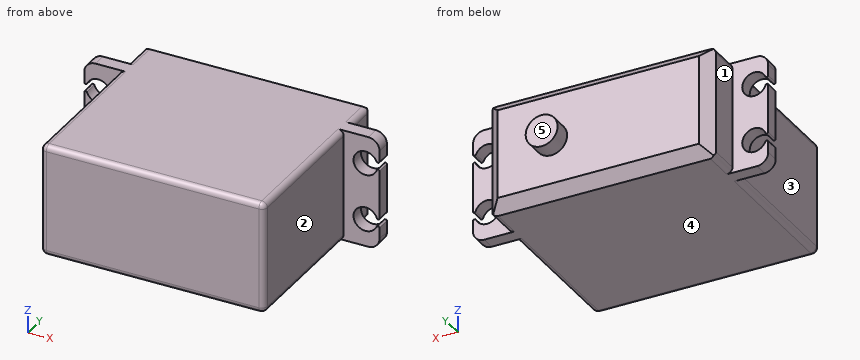
```python
from build123d import *

# Parameters (mm, degrees)
SKETCH_1_W           = 40
SKETCH_1_H           = 20
EXTRUDE_1_DEPTH      = 36.5
SKETCH_2_W           = 52.8
SKETCH_2_H           = 20
EXTRUDE_2_DEPTH      = 2.5
SKETCH_3_R           = 2.15
CUT_EXTRUDE_1_DEPTH  = 4.15
SKETCH_4_W           = 1.589858097
SKETCH_4_H           = 1.269072198
CUT_EXTRUDE_2_DEPTH  = 4.15
FILLET_2_R           = 2
FILLET_3_R           = 1
FILLET_7_R           = 0.2
FILLET_8_R           = 0.2
FILLET_START         = 38.537319575
FILLET_3_2_OUTLINE_W = 42
FILLET_3_2_OUTLINE_H = 6
FILLET_3_2_DEPTH     = 2.462680425
FILLET_START_2       = 24.395183951
FILLET_4_OUTLINE_W   = 42
FILLET_4_OUTLINE_H   = 6
FILLET_4_DEPTH       = 2.604816049
FILLET_START_3       = 52.679455198
FILLET_5_OUTLINE_W   = 5
FILLET_5_OUTLINE_H   = 22
FILLET_5_DEPTH       = 2.320544802
FILLET_START_4       = -27
FILLET_6_OUTLINE_W   = 6
FILLET_6_OUTLINE_H   = 22
FILLET_6_DEPTH       = 2.604816049
SKETCH_5_R           = 2.85
EXTRUDE_3_DEPTH      = 5
CUT_EXTRUDE_START    = -1.8
SKETCH_6_R           = 2.85
CUT_EXTRUDE_3_DEPTH  = 1.8


with BuildPart() as part:
    # 草图1 → 凸台-拉伸1 (new body)
    with BuildSketch(Plane(origin=(0, 0, 0), x_dir=(1, 0, 0), z_dir=(0, 1, 0))):
        with Locations((20, 10)):
            Rectangle(SKETCH_1_W, SKETCH_1_H)
    extrude(amount=EXTRUDE_1_DEPTH)

    # 草图2 → 凸台-拉伸2 (add)
    with BuildSketch(Plane(origin=(0, 26.5, 0), x_dir=(-1, 0, 0), z_dir=(0, -1, 0))):
        with Locations((-20, 10)):
            Rectangle(SKETCH_2_W, SKETCH_2_H)
    extrude(amount=-EXTRUDE_2_DEPTH)

    # 草图3 → 切除-拉伸1 (cut)
    with BuildSketch(Plane(origin=(0, 29, 0), x_dir=(1, 0, 0), z_dir=(0, 1, 0))):
        with Locations(Location((43.9, 15.1, 0), (0, 0, 270))):
            Circle(SKETCH_3_R)
        with Locations(Location((43.9, 4.9, 0), (0, 0, 270))):
            Circle(SKETCH_3_R)
        with Locations(Location((-3.9, 15.1, 0), (0, 0, 270))):
            Circle(SKETCH_3_R)
        with Locations(Location((-3.9, 4.9, 0), (0, 0, 270))):
            Circle(SKETCH_3_R)
    extrude(amount=-CUT_EXTRUDE_1_DEPTH, mode=Mode.SUBTRACT)

    # 草图4 → 切除-拉伸2 (cut)
    with BuildSketch(Plane(origin=(0, 29, 0), x_dir=(1, 0, 0), z_dir=(0, 1, 0))):
        with Locations((-6.117219692, 15.174989867)):
            Rectangle(SKETCH_4_W, SKETCH_4_H)
        with Locations((46.117219692, 15.174989867)):
            Rectangle(SKETCH_4_W, SKETCH_4_H)
        with Locations((46.117219692, 4.825010133)):
            Rectangle(SKETCH_4_W, SKETCH_4_H)
        with Locations((-6.117219692, 4.825010133)):
            Rectangle(SKETCH_4_W, SKETCH_4_H)
    extrude(amount=-CUT_EXTRUDE_2_DEPTH, mode=Mode.SUBTRACT)

    # 圆角2
    fillet_2_edges = [part.edges().sort_by_distance(p)[0] for p in [
        (46.4, 27.75, -20),
        (-6.4, 27.75, 0),
        (46.4, 27.75, 0),
        (-6.4, 27.75, -20),
    ]]
    fillet(fillet_2_edges, radius=FILLET_2_R)

    # Fillet 3
    fillet_3_edges = [part.edges().sort_by_distance(p)[0] for p in [
        (0, 13.25, -20),
        (40, 13.25, -20),
        (40, 13.25, 0),
        (0, 13.25, 0),
        (20, 0, -20),
        (40, 0, -10),
        (20, 0, 0),
        (0, 0, -10),
        (0, 32.75, -20),
        (40, 32.75, -20),
        (40, 32.75, 0),
        (0, 32.75, 0),
    ]]
    fillet(fillet_3_edges, radius=FILLET_3_R)

    # 圆角7
    fillet_7_edges = [part.edges().sort_by_distance(p)[0] for p in [
        (46.4, 27.75, -4.190474034),
        (46.4, 27.75, -5.459546232),
        (45.97591137, 27.75, -5.459546232),
        (45.929549926, 27.75, -4.190474034),
        (45.97591137, 27.75, -14.540453768),
        (45.929549926, 27.75, -15.809525966),
        (-5.97591137, 27.75, -5.459546232),
        (-5.929549926, 27.75, -4.190474034),
        (46.4, 27.75, -15.809525966),
        (46.4, 27.75, -14.540453768),
        (-6.4, 27.75, -4.190474034),
        (-6.4, 27.75, -5.459546232),
    ]]
    fillet(fillet_7_edges, radius=FILLET_7_R)

    # 圆角8
    fillet_8_edges = [part.edges().sort_by_distance(p)[0] for p in [
        (-6.4, 27.75, -14.540453768),
        (-6.4, 27.75, -15.809525966),
        (-5.929549926, 27.75, -15.809525966),
        (-5.97591137, 27.75, -14.540453768),
    ]]
    fillet(fillet_8_edges, radius=FILLET_8_R)

    # Fillet 3 2: read off the stored shape, not the designer's step
    # Fillet 3 2 outline → Fillet 3 2 (cut)
    with BuildSketch(Plane(origin=(0, 0, 0), x_dir=(1, 0, 0), z_dir=(0, 0.707106781186547, -0.707106781186548)).offset(FILLET_START)):
        with Locations((20, -12)):
            Rectangle(FILLET_3_2_OUTLINE_W, FILLET_3_2_OUTLINE_H)
    extrude(amount=FILLET_3_2_DEPTH, mode=Mode.SUBTRACT)

    # 倒角4: read off the stored shape, not the designer's step
    # 倒角4 outline → 倒角4 (cut)
    with BuildSketch(Plane(origin=(0, 0, 0), x_dir=(1, 0, 0), z_dir=(0, 0.707106781186547, 0.707106781186548)).offset(FILLET_START_2)):
        with Locations((20, 26)):
            Rectangle(FILLET_4_OUTLINE_W, FILLET_4_OUTLINE_H)
    extrude(amount=FILLET_4_DEPTH, mode=Mode.SUBTRACT)

    # 倒角5: read off the stored shape, not the designer's step
    # 倒角5 outline → 倒角5 (cut)
    with BuildSketch(Plane(origin=(0, 0, 0), x_dir=(0.707106781186546, -0.707106781186549, 0), z_dir=(0.707106781186549, 0.707106781186546, 0)).offset(FILLET_START_3)):
        with Locations((2.5, 10)):
            Rectangle(FILLET_5_OUTLINE_W, FILLET_5_OUTLINE_H)
    extrude(amount=FILLET_5_DEPTH, mode=Mode.SUBTRACT)

    # 倒角6: read off the stored shape, not the designer's step
    # 倒角6 outline → 倒角6 (cut)
    with BuildSketch(Plane(origin=(0, 0, 0), x_dir=(0.7071067811865471, 0.707106781186548, 0), z_dir=(0.707106781186548, -0.707106781186547, 0)).offset(FILLET_START_4)):
        with Locations((26, -10)):
            Rectangle(FILLET_6_OUTLINE_W, FILLET_6_OUTLINE_H)
    extrude(amount=FILLET_6_DEPTH, mode=Mode.SUBTRACT)

    # 草图5 → 凸台-拉伸3 (add)
    with BuildSketch(Plane(origin=(0, 36.5, 0), x_dir=(1, 0, 0), z_dir=(0, 1, 0))):
        with Locations(Location((28.4, 10, 0), (0, 0, 90))):
            Circle(SKETCH_5_R)
    extrude(amount=EXTRUDE_3_DEPTH)

    # 草图6 → 切除-拉伸3 (cut)
    with BuildSketch(Plane(origin=(0, 41.5, 0), x_dir=(1, 0, 0), z_dir=(0, 1, 0)).offset(CUT_EXTRUDE_START)):
        with Locations(Location((28.4, 10, 0), (0, 0, 90))):
            Circle(SKETCH_6_R)
    extrude(amount=CUT_EXTRUDE_3_DEPTH, mode=Mode.SUBTRACT)


solid = part.part
```
Geometry: final body of the model. Coordinates: model frame, mm. Face numbers are marked on the shaded views. A direction names the side the tool comes from. Round coordinates to 2 decimals unless told otherwise and drop trailing zeros. Order: outer loops, then holes, each group sorted by start corner. A loop starts at its lowest first (then second) coordinate and runs counter-clockwise, first axis right, second up. Notation, with made-up numbers: M -6.75,8 L 24.25,8 A25 cw 24.25,28 Z; hole C 29,53 d1. An arc over 180 degrees is marked long. One line per item, written item: value.
(1) Cut plane C-C (y = 5). Return the cut outline in (x, z).
Result sheet:
outline: M 0,-19 A1 ccw 1,-20 L 39,-20 A1 ccw 40,-19 L 40,-1 A1 ccw 39,0 L 1,0 A1 ccw 0,-1 Z
(2) Cut plane D-D (x = 35.5). Return the cut outline in (y, z).
Result sheet:
outline: M 0,-19 A1 ccw 1,-20 L 34.5,-20 L 36.5,-18 L 36.5,-2 L 34.5,0 L 1,0 A1 ccw 0,-1 Z
(3) Cut plane A-A (x = 28.4). Return the cut outline in (y, z), and give its area (3 significant figures).
Result sheet:
outline: M 0,-19 A1 ccw 1,-20 L 34.5,-20 L 36.5,-18 L 36.5,-12.85 L 39.7,-12.85 L 39.7,-7.15 L 36.5,-7.15 L 36.5,-2 L 34.5,0 L 1,0 A1 ccw 0,-1 Z
area: 744 mm2
(4) Pin query (flat end, axial travel): P1, Ø6, axis at x = 18.5, z = -7, coming from the +Y side; P2, Ø5.5, axis at x = 43.9, z = -15.1, coming from the -Y side; P3, Ø6, axis at y = 32.5, z = -11.5, coming from the -X side. Return the tip coordinate at first contact, or that it passes through.
Result sheet:
P1: y = 36.5
P2: y = 26.5
P3: x = 0
(5) Cut plane B-B (z = -10). Return the cut outline in (x, y).
Result sheet:
outline: M -6.4,26.5 L 0,26.5 L 0,1 A1 ccw 1,0 L 39,0 A1 ccw 40,1 L 40,26.5 L 46.4,26.5 L 46.4,29 L 40,29 L 40,34.5 L 38,36.5 L 31.25,36.5 L 31.25,39.7 L 25.55,39.7 L 25.55,36.5 L 2,36.5 L 0,34.5 L 0,29 L -6.4,29 Z
(6) Reachability of the marked faces 1, 2, 3, 4 and 5 from +Z, -Z, +X, -X, +Y, -Y: full face, straight path, thin tool, end or side. Return the list, or none.
Result sheet:
face 1: +Z, -Z, -X, +Y
face 2: +Z, -Z, +X, -Y
face 3: +Z, -Z, -X, -Y
face 4: -Z, +X, -X, +Y, -Y
face 5: +Z, -Z, +X, -X, +Y
(7) Line query: probe 1 along Z at (x, y) = (43.9, 28.4); probe 2 along Z at (x, y) = (-3, 28); probe 3 along X at (y, z) = (33, -10). Output: solid intervals per line, ascending. Write a range as [from, to].
Result sheet:
probe 1: [-20, -17.25], [-12.95, -7.05], [-2.75, 0]
probe 2: [-20, -17.05], [-13.15, -6.85], [-2.95, 0]
probe 3: [0, 40]
